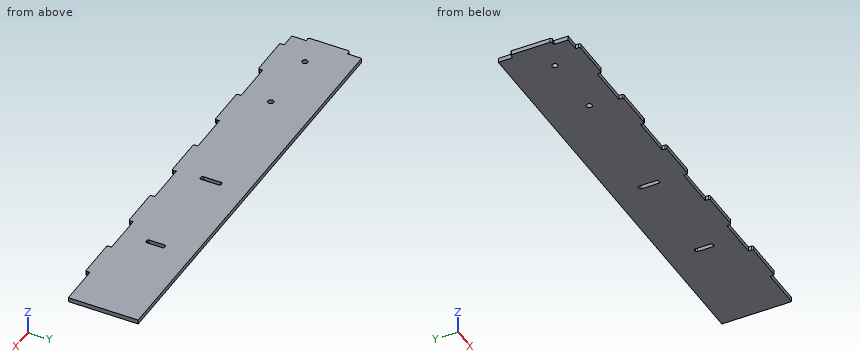
from build123d import *

# Parameters (mm, degrees)
SKETCH1_W           = 310.45
SKETCH1_H           = 50.8
BOSS_EXTRUDE1_DEPTH = 3.175
SKETCH2_R           = 2.05
SKETCH2_R_2         = 2.050488176
SKETCH2_W           = 3.175
SKETCH2_H           = 13.42251169
SKETCH2_H_2         = 15
CUT_EXTRUDE1_DEPTH  = 4.175
SKETCH3_W           = 3.175
SKETCH3_H           = 30
BOSS_EXTRUDE2_DEPTH = 3.175
SKETCH4_W           = 30
SKETCH4_H           = 3.175
BOSS_EXTRUDE3_DEPTH = 3.175
FILLET1_R           = 1


with BuildPart() as part:
    # Sketch1 → Boss-Extrude1 (new body)
    with BuildSketch(Plane.XY):
        Rectangle(SKETCH1_W, SKETCH1_H)
    extrude(amount=BOSS_EXTRUDE1_DEPTH)

    # Sketch2 → Cut-Extrude1 (cut, through all)
    with BuildSketch(Plane.XY.offset(3.175)):
        with Locations((-135.225, -5.4)):
            Circle(SKETCH2_R)
        with Locations((-87.725, -5.4)):
            Circle(SKETCH2_R_2)
        with Locations((78.9675, -1.688744155)):
            Rectangle(SKETCH2_W, SKETCH2_H)
        with Locations((3.7425, -0.9)):
            Rectangle(SKETCH2_W, SKETCH2_H_2)
    extrude(amount=-CUT_EXTRUDE1_DEPTH, mode=Mode.SUBTRACT)

    # Sketch3 → Boss-Extrude2 (add)
    with BuildSketch(Plane.ZY.offset(155.225)):
        with Locations((1.5875, 0)):
            Rectangle(SKETCH3_W, SKETCH3_H)
    extrude(amount=BOSS_EXTRUDE2_DEPTH)

    # Sketch4 → Boss-Extrude3 (add)
    with BuildSketch(Plane.XZ.offset(25.4)):
        with Locations((110.225, 1.5875)):
            Rectangle(SKETCH4_W, SKETCH4_H)
        with Locations((50.225, 1.5875)):
            Rectangle(SKETCH4_W, SKETCH4_H)
        with Locations((-9.775, 1.5875)):
            Rectangle(SKETCH4_W, SKETCH4_H)
        with Locations((-69.775, 1.5875)):
            Rectangle(SKETCH4_W, SKETCH4_H)
        with Locations((-129.775, 1.5875)):
            Rectangle(SKETCH4_W, SKETCH4_H)
    extrude(amount=BOSS_EXTRUDE3_DEPTH)

    # Fillet1
    fillet1_edges = [part.edges().sort_by_distance(p)[0] for p in [
        (-84.775, -28.575, 1.5875),
        (-54.775, -28.575, 1.5875),
        (-144.775, -28.575, 1.5875),
        (-114.775, -28.575, 1.5875),
        (80.555, 5.02251169, 1.5875),
        (80.555, -8.4, 1.5875),
        (77.38, -8.4, 1.5875),
        (77.38, 5.02251169, 1.5875),
        (5.33, 6.6, 1.5875),
        (5.33, -8.4, 1.5875),
        (2.155, -8.4, 1.5875),
        (2.155, 6.6, 1.5875),
        (-158.4, 15, 1.5875),
        (-158.4, -15, 1.5875),
        (125.225, -28.575, 1.5875),
        (95.225, -28.575, 1.5875),
        (35.225, -28.575, 1.5875),
        (65.225, -28.575, 1.5875),
        (-24.775, -28.575, 1.5875),
        (5.225, -28.575, 1.5875),
    ]]
    fillet(fillet1_edges, radius=FILLET1_R)


solid = part.part
Here's how the part is built. I have some questions about the finished solid (model axes, mm). Round coordinates to 2 decimals unless told otherwise and drop trailing zeros. Write each loop counter-clockwise with the first axis right and the second up, starting at its lowest first coordinate (ties: lowest second). Pieces come first, ordered by that corner, then holes.
1. Suppose I cut it at B-B (x = 30). List the corners of the cut face in (y, z) for me (3 decimals), and give its area (3 significant figures).
2. Suppose I cut it at A-A (z = 1.4). State how many separate pieces and enclosed holes the cut face has, and give its area (3 significant figures).
3. I need wall thicknesses on L1, parallel to X at y = 4, z = 2.35 (3 decimals); L2, parallel to Y at x = 132, z = 2.55; L3, parallel to Y at x = -89, z = 1.6. Which ranges of each line are inside material? Lowest first, please.
4. Will these pins go through, and if not, where does the flat tip stop? pin 1 Ø0.7 at (x, z) = (-156.5, 2) entering from -Y; pin 2 Ø1.7 at (y, z) = (-27, 2) entering from -X (3 decimals); pin 3 Ø1.1 at (y, z) = (-27, 1.5) entering from +X (3 decimals).
Answer sheet:
1. outline: (-25.4, 0) - (25.4, 0) - (25.4, 3.175) - (-25.4, 3.175) - close
1. area: 161 mm2
2. separate pieces: 1
2. enclosed holes: 4
2. area: 16,200 mm2
3. L1: x = -158.4 to 2.155, 5.33 to 77.38, 80.555 to 155.225
3. L2: y = -25.4 to 25.4
3. L3: y = -25.4 to -7.01, -3.79 to 25.4
4. pin 1: stops at y = -15
4. pin 2: stops at x = -144.775
4. pin 3: stops at x = 125.225
